Geometry check sheet. Reference: drawing and pictorial views, mm from the part's lowest x, y, z. A direction names the side the tool comes from. Round coordinates to 2 decimals unless told otherwise and drop trailing zeros. Order: outer loops, then holes, each group sorted by start corner. A loop starts at its lowest first (then second) coordinate and runs counter-clockwise, first axis right, second up.
(1) Gauge pin test, flat ends, axial feed: P1, Ø4, axis at x = 2, y = 4.5, coming from the -Z side; P2, Ø3.5, axis at x = 5, z = 5.5, coming from the +Y side; P3, Ø4, axis at x = 8.5, y = 19, coming from the +Z side; P4, Ø1.8, axis at x = 7, y = 19, coming from the -Z side. Record the tip position at first contact, or that the pin passes through.
(2) Cross-section at D-D on z = 11.25. Enter the section's corners in (x, y).
(3) Set-up check for the marked faces 4, 5, 6 and 7: record each of +Z, -Z, +X, -X, +Y, -Y from which the full face is reachable in a straight line by a thin tool's end or side.
(4) Thickness scan on L1, parallel to Y at x = 6.25, z = 7.25; L2, parallel to Z at x = 8.75, y = 20; L3, parallel to X at y = 19.5, z = 7.7. Record the ranges inside material, lowest first.
(5) Cross-section at C-C on x = 3.75. Enter the section's corners in (y, z), and give its area (3 significant figures).
(6) Cross-section at A-A on y = 19.5. Enter the section's corners in (x, z), and give its area (3 significant figures).
(7) Cross-section at B-B on x = 6.25. Enter the section's corners in (y, z).
(8) Draft check along X on the marked faces 1, 2 and 3. Enter one of: pulls with the +X half, pulls with the -X half, needs draft (parallel to the pull), parting line crosses it, or undercut.
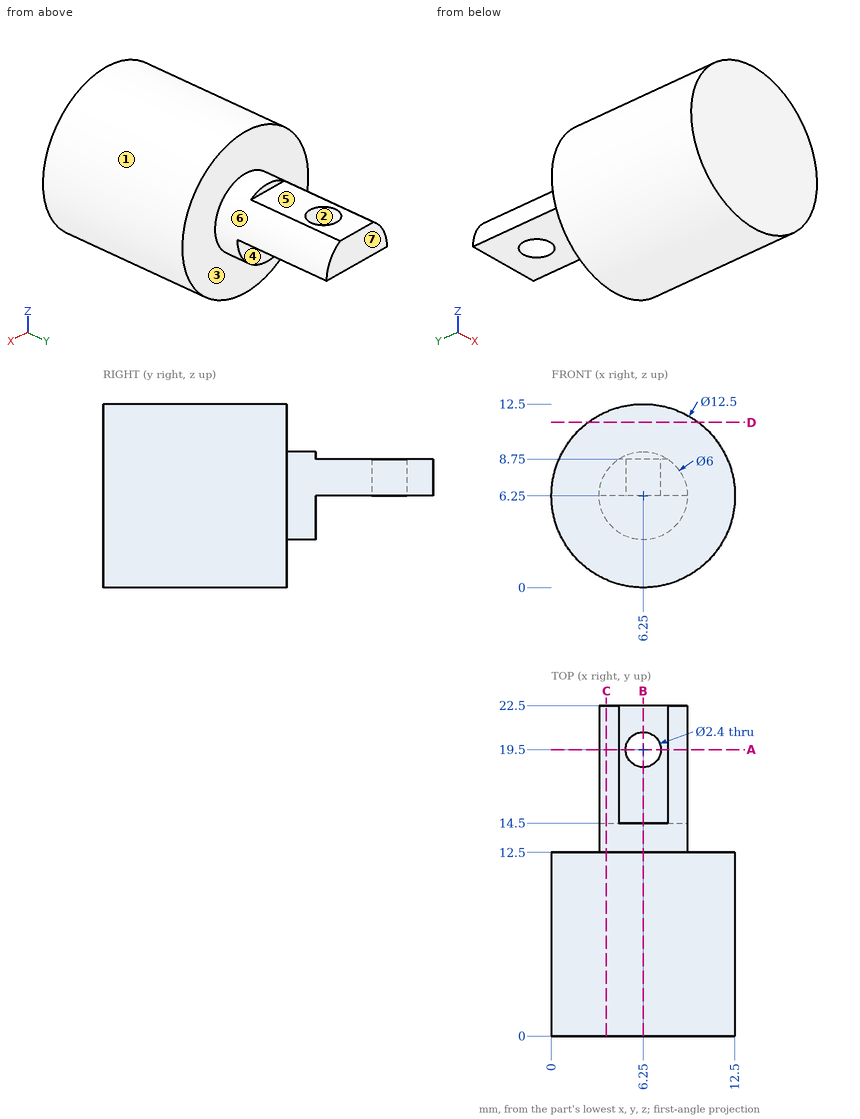
Found:
1. P1: stops at z = 0.42
1. P2: stops at y = 22.5
1. P3: stops at z = 8.75
1. P4: stops at z = 6.25
2. outline: (2.5, 0) - (10, 0) - (10, 12.5) - (2.5, 12.5) - close
3. face 4: -Z, +X, -X, +Y
3. face 5: +Z, +X, -X, +Y
3. face 6: +Y
3. face 7: +Z, -Z, +X, -X, +Y
4. L1: y = 0 to 18.3, 20.7 to 22.5
4. L2: z = 6.25 to 7.91
4. L3: x = 3.62 to 5.05, 7.45 to 8.88
5. outline: (0, 0.52) - (12.5, 0.52) - (12.5, 4.59) - (14.5, 4.59) - (14.5, 6.25) - (22.5, 6.25) - (22.5, 7.91) - (12.5, 7.91) - (12.5, 11.98) - (0, 11.98) - close
5. area: 163 mm2
6. outline: (3.25, 6.25) - (5.05, 6.25) - (5.05, 8.75) - (4.59, 8.75) arc R3 ccw to start; (7.45, 6.25) - (9.25, 6.25) arc R3 ccw to (7.91, 8.75) - (7.45, 8.75) - close
6. area: 7.01 mm2
7. outline: (0, 0) - (12.5, 0) - (12.5, 3.25) - (14.5, 3.25) - (14.5, 6.25) - (18.3, 6.25) - (18.3, 8.75) - (14.5, 8.75) - (14.5, 9.25) - (12.5, 9.25) - (12.5, 12.5) - (0, 12.5) - close; (20.7, 6.25) - (22.5, 6.25) - (22.5, 8.75) - (20.7, 8.75) - close
8. face 1: parting line crosses it
8. face 2: undercut
8. face 3: needs draft
